Study the drawing (mm; zero at the part's minimum x, y, z) and answer. A direction names the side the tool comes from. Coordinates: 2 decimals unless noted, no trailing zeros. Write each loop counter-clockwise with the first axis right and the second up, starting at its lowest first coordinate (ties: lowest second). Pieces come first, ordered by that corner, then holes. Notation, with made-up numbers: (-39.5, 47) -> (-19.5, 47) arc R36 cw to (-19.5, 82) -> close; hole circle Ø9 at (61.25, -32). An arc over 180 degrees is marked (long way). Write item = value, one per line. Start each with the question number.
1) Find the intervals of material crossed by line 1 along Z through (x, y) = (5.5, 7.5); line 2 along Y through (x, z) = (2.5, 7.75); line 3 along Z through (x, y) = (5.5, 5), in increasing order. Write a range as from..to.
2) Section B-B (x = 3) is taken. Determine the outline of the cut face in (y, z).
3) A tool of negligible diameter and unlimited length cuts with its end or side. For the marked faces 1, 2, 3, 4 and 5, from which of +Z, -Z, +X, -X, +Y, -Y can it reach the whole face along a straight path? Write none if from no direction.
4) Section C-C (z = 5) is taken. Determine the outline of the cut face in (x, y).
5) Section A-A (z = 7.5) is taken. Determine the outline of the cut face in (x, y).
6) For a pull along Z with two mould halves and no side action, classify the marked faces 6, 7, 8 and 9 as released by +Z, released by -Z, zero draft, split by the parting line, or undercut.
7) Flat-ended cylindrical pins translate along their axes: pin 1 Ø3 at (y, z) = (7.5, 10.5) entering from -X; pin 2 Ø5 at (y, z) = (3.5, 3) entering from -X; pin 3 Ø2.5 at (x, y) = (3, 2) entering from -Z; pin 4 Ø1.5 at (x, y) = (2.5, 4.5) entering from +Z. Find the tip coordinate at first contact, or state that the pin passes through.
8) Section D-D (z = 2.25) is taken. Determine the outline of the cut face in (x, y).
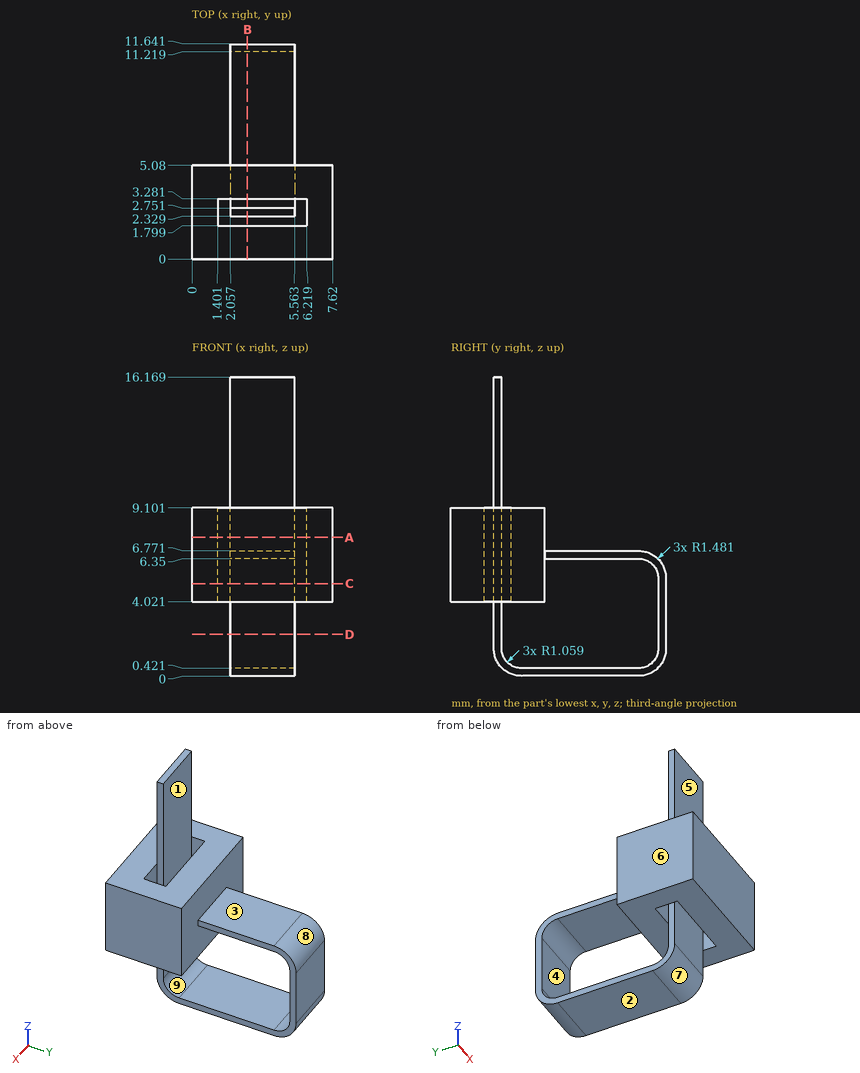
Answer key:
q1.line_1 = 0..0.42, 6.35..6.77
q1.line_2 = 0..1.8, 2.33..2.75, 3.28..5.08
q1.line_3 = 0..0.42, 4.02..9.1
q2.outline = (0, 4.02) -> (1.8, 4.02) -> (1.8, 9.1) -> (0, 9.1) -> close; (2.33, 1.48) arc R1.48 ccw to (3.81, 0) -> (10.16, 0) arc R1.48 ccw to (11.64, 1.48) -> (11.64, 5.29) arc R1.48 ccw to (10.16, 6.77) -> (5.08, 6.77) -> (5.08, 9.1) -> (3.28, 9.1) -> (3.28, 4.02) -> (5.08, 4.02) -> (5.08, 6.35) -> (10.16, 6.35) arc R1.06 cw to (11.22, 5.29) -> (11.22, 1.48) arc R1.06 cw to (10.16, 0.42) -> (3.81, 0.42) arc R1.06 cw to (2.75, 1.48) -> (2.75, 16.17) -> (2.33, 16.17) -> close
q3.face_1 = +Z
q3.face_2 = -Z, +X, -X, +Y, -Y
q3.face_3 = +Z, +X, -X, +Y
q3.face_4 = +X, -X
q3.face_5 = +Z, -Z
q4.outline = (0, 0) -> (7.62, 0) -> (7.62, 5.08) -> (0, 5.08) -> close; (2.06, 2.33) -> (5.56, 2.33) -> (5.56, 2.75) -> (2.06, 2.75) -> close; (2.06, 11.22) -> (5.56, 11.22) -> (5.56, 11.64) -> (2.06, 11.64) -> close; hole (1.4, 1.8) -> (6.22, 1.8) -> (6.22, 3.28) -> (1.4, 3.28) -> close
q5.outline = (0, 0) -> (7.62, 0) -> (7.62, 5.08) -> (0, 5.08) -> close; (2.06, 2.33) -> (5.56, 2.33) -> (5.56, 2.75) -> (2.06, 2.75) -> close; hole (1.4, 1.8) -> (6.22, 1.8) -> (6.22, 3.28) -> (1.4, 3.28) -> close
q6.face_6 = zero draft
q6.face_7 = released by -Z
q6.face_8 = released by +Z
q6.face_9 = undercut
q7.pin_1 = through
q7.pin_2 = 0
q7.pin_3 = 0.11
q7.pin_4 = 9.1
q8.outline = (2.06, 2.33) -> (5.56, 2.33) -> (5.56, 2.75) -> (2.06, 2.75) -> close; (2.06, 11.22) -> (5.56, 11.22) -> (5.56, 11.64) -> (2.06, 11.64) -> close
